Geometry check sheet. Reference: the model listing, model coordinates, mm. Face numbers are marked on the shaded views. A direction names the side the tool comes from. Give positions to 0.01 mm unless a question says otherwise; leave off trailing zeros. Order: outer loops, then holes, each group sorted by start corner. A loop starts at its lowest first (then second) coordinate and runs counter-clockwise, first axis right, second up.
from build123d import *


with BuildPart() as part:
    # Sketch1 → Revolve3 (revolve)
    with BuildSketch(Plane(origin=(0, 0, 0), x_dir=(1, 0, 0), z_dir=(0, 1, 0))):
        with BuildLine():
            Line((0, 0), (0, 230))
            Line((0, 230), (12.5, 230))
            Line((12.5, 230), (12.5, 218))
            Line((12.5, 218), (14, 217.999999999))
            Line((14, 217.999999999), (13.999927666, 216))
            Line((13.999927666, 216), (12.515611153, 216))
            Line((12.515611153, 216), (12.5, 210.98853812))
            Line((12.5, 210.98853812), (15.499978569, 210.999877804))
            Line((15.499978569, 210.999877804), (15.515611153, 210))
            Line((15.515611153, 210), (12.5, 210))
            add(Edge.make_bspline(
                [(12.5, 210), (14.922130771, 175.127506462), (31.979338754, 179.564350306), (32.5, 145)],
                knots=[0, 0, 0, 0, 1, 1, 1, 1], degree=3))
            Line((32.5, 145), (32.5, 90))
            add(Edge.make_bspline(
                [(32.5, 90), (25.721809169, 83.316192042), (26.936513276, 82.414233108), (26.810048481, 66.997733089), (28.46817148, 57.131214713), (32.096286638, 44.010772021), (34.987931681, 23.776222362), (33.214929298, 10.739901), (27.5, 0)],
                knots=[0, 0, 0, 0, 0.249131323, 0.300005802, 0.485551569, 0.527189357, 0.693190465, 1, 1, 1, 1], degree=3))
            Line((27.5, 0), (0, 0))
        make_face()
    revolve(axis=Axis((0, 0, 0), (0, 0, -1)))


solid = part.part
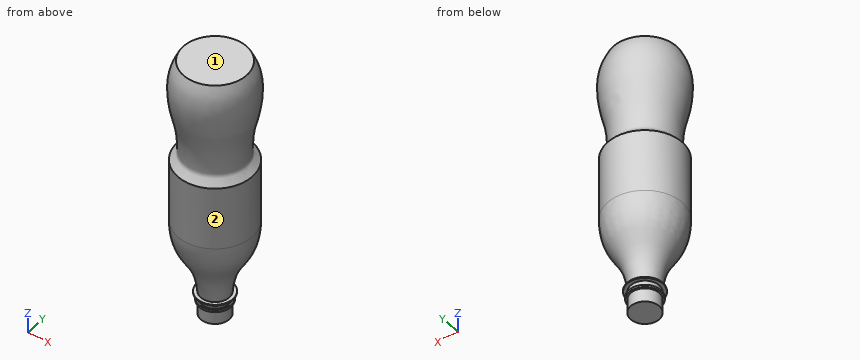
Item 1: Gauge pin test, flat ends, axial feed: pin 1 (5 mm diameter, centred on y = 15, z = -36.5, fed in from -X); pin 2 (6 mm diameter, centred on x = 23.5, z = -90, fed in from -Y); pin 3 (6 mm diameter, centred on x = -10.5, z = -183, fed in from -Y). Record the tip position at first contact, or that the pin passes through.
Reported:
pin 1: stops at x = -30.62
pin 2: stops at y = -25.22
pin 3: stops at y = -19.4
Item 2: Scan lines: L1, parallel to X at y = 1, z = -218.5; L2, parallel to X at y = -21, z = -108; L3, parallel to Y at x = -9, z = -15. Record each from-to range of solid material in increasing order.
Reported:
L1: x = -12.46 to 12.46
L2: x = -24.8 to 24.8
L3: y = -31.74 to 31.74
Item 3: Sectioned sample at A-A (z = -142). Enter the section's corners in (x, y), and give its area (3 significant figures).
Reported:
outline: circle Ø65 at (0, 0)
area: 3,320 mm2
Item 4: Set-up check for the marked faces 1 and 2: record each of +Z, -Z, +X, -X, +Y, -Y from which the full face is reachable in a straight line by a thin tool's end or side.
Reported:
face 1: +Z, +X, -X, +Y, -Y
face 2: -Z
